from build123d import *

# Parameters (mm, degrees)
F1_DEPTH = 160


with BuildPart() as f1:
    # F0 (on Top) → F1 (new body)
    with BuildSketch(Plane.XY):
        Polygon((-4, 16.818339), (0, 16.818339), (1835, 16.818339), (1839, 16.818339), (1839, 20.818339), (1429, 730.818339), (1429, 734.818339), (1426.690141, 734.818339), (1425, 734.818339), (0, 734.818339), (-4, 734.818339), (-4, 730.818339), (-4, 20.818339), align=None)
        Polygon((1835, 20.818339), (0, 20.818339), (0, 730.818339), (1425, 730.818339), align=None, mode=Mode.SUBTRACT)
    extrude(amount=F1_DEPTH)


solid = f1.part
Source: CAD feature listing. Evaluate the final solid. Frame: model axes, mm. A direction names the side the tool comes from. Coordinates: 2 decimals unless noted, no trailing zeros. Loops run counter-clockwise (first coordinate to the right, second up) from the corner with the lowest first, then second, coordinate; pieces in that order, holes last. Notation, with made-up numbers: (30, 70.25) - (39, 70.25) arc R33 cw to (39, 106.25) - close; hole circle Ø9 at (71.5, 66). An arc over 180 degrees is marked (long way). One line per item, written item: value. Start each with the question number.
1. Section C-C (y = 315). Return the cut outline in (x, z), and give its area (3 significant figures).
2. Mould query, pull axis Y, two halves, no side actions, for faces 3 (the flat face through (905, 16.818, 79)), 4 (the flat face through (1627.13, 380.79, 78.88)), 5 (the flat face through (1636.9, 370.8, 78.9)), 6 (the flat face through (-4, 381, 79)). Classes: pulls with the +Y half, pulls with the -Y half, needs draft (parallel to the pull), parting line crosses it, or undercut.
3. Set-up query: faces 1 (the flat face through (703, 730.818, 79)), 2 (the flat face through (723, 734.818, 79)). Return all of +Z, -Z, +X, -X, +Y, -Y with unobstructed straight access to the full face (end or side cutting, diameter ignored); none if empty.
4. Section A-A (x = 179). Return the cut outline in (y, z).
5. Contact query for flat-ended pins moving along their axis: P1, Ø1, axis at y = 295, z = 113, coming from the +X side; P2, Ø1.2, axis at y = 733, z = 46, coming from the +X side; P3, Ø6, axis at x = 1623.5, z = 45, coming from the +Y side. Output: stop coordinate, or through.
6. Ray query, L1, parallel to Y at x = 360, z = 143.5; L2, parallel to X at y = 295.5, z = 84; L3, parallel to X at y = 701, z = 33. Return the intervals inside material, ascending.
7. Section B-B (z = 92). Return the cut outline in (x, y), and give its area (3 significant figures).
Verdict:
1. outline: (-4, 0) - (0, 0) - (0, 160) - (-4, 160) - close; (1665.12, 0) - (1669.12, 0) - (1669.12, 160) - (1665.12, 160) - close
1. area: 1,280 mm2
2. face 3: pulls with the -Y half
2. face 4: undercut
2. face 5: pulls with the +Y half
2. face 6: needs draft
3. face 1: +Z, -Z
3. face 2: +Z, -Z, +X, -X, +Y
4. outline: (16.82, 0) - (20.82, 0) - (20.82, 160) - (16.82, 160) - close; (730.82, 0) - (734.82, 0) - (734.82, 160) - (730.82, 160) - close
5. P1: stops at x = 1680.96
5. P2: stops at x = 1429
5. P3: stops at y = 399.2
6. L1: y = 16.82 to 20.82, 730.82 to 734.82
6. L2: x = -4 to 0, 1676.38 to 1680.38
6. L3: x = -4 to 0, 1442.22 to 1446.22
7. outline: (-4, 16.82) - (1839, 16.82) - (1839, 20.82) - (1429, 730.82) - (1429, 734.82) - (-4, 734.82) - close; hole (0, 20.82) - (1835, 20.82) - (1425, 730.82) - (0, 730.82) - close
7. area: 18,800 mm2
